```python
from build123d import *

# Parameters (mm, degrees)
SKETCH_1_W                = 65
SKETCH_1_H                = 250
EXTRUDE_1_DEPTH           = 10
HOLE_WIZARD_1_D           = 5.5
HOLE_WIZARD_1_DEPTH       = 18
HOLE_WIZARD_1_CBORE_D     = 10
HOLE_WIZARD_1_CBORE_DEPTH = 5.7
HOLE_WIZARD_1_TIP         = 1.652366702
HOLE_WIZARD_M6_1_D        = 5
HOLE_WIZARD_M6_1_DEPTH    = 17
HOLE_WIZARD_M6_1_TIP      = 1.502151548


with BuildPart() as part:
    # 草图1 → 凸台-拉伸1 (new body)
    with BuildSketch(Plane.XY):
        Rectangle(SKETCH_1_W, SKETCH_1_H)
    extrude(amount=EXTRUDE_1_DEPTH)

    # 打孔尺寸(%根据)内六角圆柱头螺钉的类型1
    with Locations(Plane(origin=(-6.5, 107, 0), x_dir=(-1, 0, 0), z_dir=(0, 0, -1))):
        with Locations((0, 0), (-32, 0), (0, -36), (-32, -36), (-32, -178), (0, -178), (0, -214), (-32, -214)):
            CounterBoreHole(HOLE_WIZARD_1_D / 2, HOLE_WIZARD_1_CBORE_D / 2, HOLE_WIZARD_1_CBORE_DEPTH, depth=HOLE_WIZARD_1_DEPTH)
            with Locations((0, 0, -(HOLE_WIZARD_1_DEPTH + HOLE_WIZARD_1_TIP / 2))):  # 118° drill point
                Cone(0, HOLE_WIZARD_1_D / 2, HOLE_WIZARD_1_TIP, mode=Mode.SUBTRACT)

    # M6 螺纹孔1
    with Locations(Plane(origin=(-32.5, -70, 5), x_dir=(0, -1, 0), z_dir=(-1, 0, 0))):
        with Locations((0, 0), (-35, 0), (-70, 0), (-105, 0), (-140, 0), (35, 0), (-175, 0)):
            Hole(HOLE_WIZARD_M6_1_D / 2, depth=HOLE_WIZARD_M6_1_DEPTH)
            with Locations((0, 0, -(HOLE_WIZARD_M6_1_DEPTH + HOLE_WIZARD_M6_1_TIP / 2))):  # 118° drill point
                Cone(0, HOLE_WIZARD_M6_1_D / 2, HOLE_WIZARD_M6_1_TIP, mode=Mode.SUBTRACT)


solid = part.part
```
CAD build for the part. Positions are in the model's coordinates, mm. A direction names the side the tool comes from. Round coordinates to 2 decimals unless told otherwise and drop trailing zeros. Order: outer loops, then holes, each group sorted by start corner. A loop starts at its lowest first (then second) coordinate and runs counter-clockwise, first axis right, second up.
Q1. Which spindle directions (+Z, -Z, +X, -X, +Y, -Y) get a long thin tool onto all of the face, cutting with end or side? Do faces 1 (the cylindrical face through (25.142, -68.273, 7.88)), 2 (the cylindrical face through (-23.881, -102.615, 5.751)), 3 (the cylindrical face through (-9.188, -66.784, 2.81)). Say none if no direction does.
Q2. Slice it at A-A (x = -18). Write the cut outline in (y, z), and give its area (3 significant figures).
Q3. Two-plate mould, pull along X, no slides. Class faces 4 (the cylindrical face through (24.904, 104.315, 7.88)), 5 (the conical face through (-14, 0, 5)), 6 (the flat face through (0, 2, 0)): pulls with the +X half, pulls with the -X half, needs draft (parallel to the pull), parting line crosses it, or undercut.
Q4. Wall check: L1, parallel to Y at x = 25.5, z = 3.75; L2, parallel to Y at x = -11, z = 3.5; L3, parallel to X at y = 109, z = 1.5. Give the ranges that are in metal, low to high.
Q5. Drop a flat-ended pin along its axis: pin 1 (3 mm diameter, centred on x = 25, y = 109.5, fed in from -Z). Give the stop position or say it passes through.
Results below:
1. face 1: +Z, -Z
1. face 2: -X
1. face 3: -Z
2. outline: (-125, 0) - (125, 0) - (125, 10) - (-125, 10) - close; hole circle Ø5 at (-105, 5); hole circle Ø5 at (-70, 5); hole circle Ø5 at (-35, 5); hole circle Ø5 at (0, 5); hole circle Ø5 at (35, 5); hole circle Ø5 at (70, 5); hole circle Ø5 at (105, 5)
2. area: 2,360 mm2
3. face 4: undercut
3. face 5: pulls with the -X half
3. face 6: needs draft
4. L1: y = -125 to -112, -102 to -76, -66 to 66, 76 to 102, 112 to 125
4. L2: y = -125 to -109.18, -104.82 to -73.18, -68.82 to 68.82, 73.18 to 104.82, 109.18 to 125
4. L3: x = -32.5 to -11.08, -1.92 to 20.92, 30.08 to 32.5
5. pin 1: stops at z = 5.7
